Check sheet for the modelled part. Datum: model origin and axes. Units: mm. Give positions to 0.01 mm unless a question says otherwise; leave off trailing zeros. Write each loop counter-clockwise with the first axis right and the second up, starting at its lowest first coordinate (ties: lowest second). Pieces come first, ordered by that corner, then holes. Notation, with made-up numbers: (82.25, -1.75) -> (123.25, -1.75) arc R18 ccw to (123.25, 17.25) -> close; hole circle Ø6 at (84.25, -28.75). An arc over 180 degrees is marked (long way). Write each question's results on one line, items separated by ' | '. Start each with the question number.
```python
from build123d import *

# Parameters (mm, degrees)
ESQUISSE1_W               = 320
ESQUISSE1_H               = 120
BOSS_EXTRU_1_DEPTH        = 6
M25_CLEARANCE_HOLE1_D     = 27
M25_CLEARANCE_HOLE1_DEPTH = 6
M25_CLEARANCE_HOLE1_TIP   = 8.111618357


with BuildPart() as part:
    # Esquisse1 → Boss.-Extru.1 (new body)
    with BuildSketch(Plane.XY):
        Rectangle(ESQUISSE1_W, ESQUISSE1_H)
    extrude(amount=BOSS_EXTRU_1_DEPTH)

    # M25 Clearance Hole1
    with Locations(Plane.XY.offset(6)):
        with Locations((-103.53808412, 0), (0, 0), (84.253962724, 0)):
            Hole(M25_CLEARANCE_HOLE1_D / 2, depth=M25_CLEARANCE_HOLE1_DEPTH)
            with Locations((0, 0, -(M25_CLEARANCE_HOLE1_DEPTH + M25_CLEARANCE_HOLE1_TIP / 2))):  # 118° drill point
                Cone(0, M25_CLEARANCE_HOLE1_D / 2, M25_CLEARANCE_HOLE1_TIP, mode=Mode.SUBTRACT)


solid = part.part
```
Item 1: Section check A-A on y = 0. Record the boundary of the cut face in (x, z), then the cut area to 3 significant figures.
Item 2: Section check C-C on z = 4.75. Record the boundary of the cut face in (x, y).
Item 3: Section check B-B on x = 0. Record the boundary of the cut face in (y, z).
Item 4: Thickness scan on probe 1 along X at (y, z) = (0, 4.8); probe 2 along Y at (x, z) = (0, 4); probe 3 along Y at (x, z) = (94.5, 5.3). Record the ranges inside material, lowest first. Write a range as from..to.
Item 5: Mould release check, pull along Y, two halves, no side actions. Record for faces 1 (the flat face through (-160, -1, 3)), 2 (the flat face through (-2, 60, 3)), 3 (the flat face through (-2, -60, 3)), 4 (the cylindrical face through (-116.01, -5.17, 2.96)): pulls with the +Y half, pulls with the -Y half, needs draft (parallel to the pull), parting line crosses it, or undercut.
Check sheet entries:
1) outline: (-160, 0) -> (-117.04, 0) -> (-117.04, 6) -> (-160, 6) -> close; (-90.04, 0) -> (-13.5, 0) -> (-13.5, 6) -> (-90.04, 6) -> close; (13.5, 0) -> (70.75, 0) -> (70.75, 6) -> (13.5, 6) -> close; (97.75, 0) -> (160, 0) -> (160, 6) -> (97.75, 6) -> close | area: 1,430 mm^2
2) outline: (-160, -60) -> (160, -60) -> (160, 60) -> (-160, 60) -> close; hole circle Ø27 at (-103.54, 0); hole circle Ø27 at (0, 0); hole circle Ø27 at (84.25, 0)
3) outline: (-60, 0) -> (-13.5, 0) -> (-13.5, 6) -> (-60, 6) -> close; (13.5, 0) -> (60, 0) -> (60, 6) -> (13.5, 6) -> close
4) probe 1: x = -160..-117.04, -90.04..-13.5, 13.5..70.75, 97.75..160 | probe 2: y = -60..-13.5, 13.5..60 | probe 3: y = -60..-8.79, 8.79..60
5) face 1: needs draft | face 2: pulls with the +Y half | face 3: pulls with the -Y half | face 4: undercut
